```python
from build123d import *

# Parameters (mm, degrees)
SKETCH_1_W           = 29.5
SKETCH_1_H           = 47
EXTRUDE_1_DEPTH      = 70
SKETCH_2_W           = 23.5
SKETCH_2_H           = 44
CUT_EXTRUDE_1_DEPTH  = 70
SKETCH_5_R           = 12
SKETCH_5_R_2         = 3
CUT_EXTRUDE_4_DEPTH  = 70
SKETCH_10_R          = 9
CUT_EXTRUDE_8_DEPTH  = 17
SKETCH_11_W          = 23.5
SKETCH_11_H          = 26.5
SKETCH_11_H_2        = 15
CUT_EXTRUDE_9_DEPTH  = 10
FILLET_2_R           = 5
CUT_EXTRUDE_11_DEPTH = 10
FILLET_3_R           = 5
SKETCH_14_R          = 1.5
CUT_EXTRUDE_12_DEPTH = 10


with BuildPart() as part:
    # 草图1 → 凸台-拉伸1 (new body)
    with BuildSketch(Plane.XY):
        with Locations((14.75, 23.5)):
            Rectangle(SKETCH_1_W, SKETCH_1_H)
    extrude(amount=EXTRUDE_1_DEPTH)

    # 草图2 → 切除-拉伸1 (cut)
    with BuildSketch(Plane.XY.offset(70)):
        with Locations((14.75, 25)):
            Rectangle(SKETCH_2_W, SKETCH_2_H)
    extrude(amount=-CUT_EXTRUDE_1_DEPTH, mode=Mode.SUBTRACT)

    # 草图5 → 切除-拉伸4 (cut)
    with BuildSketch(Plane(origin=(29.5, 0, 0), x_dir=(0, 0, -1), z_dir=(1, 0, 0))):
        with Locations((-17, 32)):
            Circle(SKETCH_5_R)
        with Locations((-62, 32)):
            Circle(SKETCH_5_R_2)
    extrude(amount=-CUT_EXTRUDE_4_DEPTH, mode=Mode.SUBTRACT)

    # 草图10 → 切除-拉伸8 (cut)
    with BuildSketch(Plane(origin=(29.5, 0, 0), x_dir=(0, 0, -1), z_dir=(1, 0, 0))):
        with Locations((-45, 16)):
            Circle(SKETCH_10_R)
    extrude(amount=-CUT_EXTRUDE_8_DEPTH, mode=Mode.SUBTRACT)

    # 草图11 → 切除-拉伸9 (cut)
    with BuildSketch(Plane.XZ):
        with Locations((14.75, 56.75)):
            Rectangle(SKETCH_11_W, SKETCH_11_H)
        with Locations((14.75, 7.5)):
            Rectangle(SKETCH_11_W, SKETCH_11_H_2)
    extrude(amount=-CUT_EXTRUDE_9_DEPTH, mode=Mode.SUBTRACT)

    # 圆角2
    fillet_2_edges = [part.edges().sort_by_distance(p)[0] for p in [
        (1.5, 0, 0),
        (28, 0, 0),
        (28, 0, 70),
        (1.5, 0, 70),
        (3, 1.5, 43.5),
        (26.5, 1.5, 43.5),
    ]]
    fillet(fillet_2_edges, radius=FILLET_2_R)

    # 草图13 → 切除-拉伸11 (cut)
    with BuildSketch(Plane(origin=(3, 0, 0), x_dir=(0, 0, -1), z_dir=(1, 0, 0))):
        Polygon((-15, 0), (-15, 3), (-30, 3), (-56, 47), (0, 47), (0, 0), align=None)
    extrude(amount=-CUT_EXTRUDE_11_DEPTH, mode=Mode.SUBTRACT)

    # 圆角3
    fillet_3_edges = [part.edges().sort_by_distance(p)[0] for p in [
        (28, 47, 70),
        (0, 1.5, 15),
        (1.5, 3, 30),
        (1.5, 47, 56),
        (1.5, 47, 70),
        (28, 47, 0),
        (26.5, 1.5, 15),
    ]]
    fillet(fillet_3_edges, radius=FILLET_3_R)

    # 草图14 → 切除-拉伸12 (cut)
    with BuildSketch(Plane.XZ):
        with Locations(Location((9.75, 35.2, 0), (0, 0, 270))):
            Circle(SKETCH_14_R)
        with Locations(Location((9.75, 23.2, 0), (0, 0, 270))):
            Circle(SKETCH_14_R)
        with Locations(Location((19.75, 23.2, 0), (0, 0, 270))):
            Circle(SKETCH_14_R)
        with Locations(Location((19.75, 35.2, 0), (0, 0, 270))):
            Circle(SKETCH_14_R)
    extrude(amount=-CUT_EXTRUDE_12_DEPTH, mode=Mode.SUBTRACT)


solid = part.part
```
The listing builds one solid part. Answer for the finished solid, in the listing's coordinates (mm). A direction names the side the tool comes from. Coordinates: 2 decimals unless noted, no trailing zeros. Loops run counter-clockwise (first coordinate to the right, second up) from the corner with the lowest first, then second, coordinate; pieces in that order, holes last. Notation, with made-up numbers: (-17, -7) -> (11, -7) arc R16 cw to (11, 4) -> close; hole circle Ø4 at (63.5, 15.25). An arc over 180 degrees is marked (long way). Return JSON: item names as keys, results as strings. Group by question number.
(1) A cutting plane is placed at B-B on x = 19.75. Write down the section's boundary in (y, z).
(2) A cutting plane is placed at D-D on y = 36. Write down the section's boundary in (x, z).
(3) A cutting plane is placed at C-C on z = 35.2. Write down the section's boundary in (x, y), and give its area (3 significant figures).
(4) A cutting plane is placed at A-A on z = 62. Write down the section's boundary in (x, y).
(5) Determine the mould class of faces 6 (the cylindrical face through (28, 46, 2)), 7 (the cylindrical face through (28, 2, 1)), 8 (the cylindrical face through (1.5, 30.2, 64.4)) for opening direction Y: released by +Y, released by -Y, zero draft, split by the parting line, or undercut.
(6) Which of the six approach directions +Z, -Z, +X, -X, +Y, -Y give full straight-line access (tool end or side, diameter ignored) to faces 1 (the cylindrical face through (28, 16, 54)), 2 (the cylindrical face through (21.237, 1.479, 23.395)), 3 (the cylindrical face through (28, 2, 69)), 4 (the flat face through (2, 25, 43)), 5 (the flat face through (15, 1, 43.5))?
(7) Find the intervals of material crossed by probe 1 along X at (y, z) = (1, 35.2); probe 2 along X at (y, z) = (13, 60.5); probe 3 along Y at (x, z) = (27.6, 62), in increasing order. Write a range as from..to.
(8) Given pin 1 Ø13 at (x, z) = (14, 33) entering from +Y; pin 2 Ø2.5 at (x, y) = (16.5, 2) entering from -Z; pin 3 Ø3 at (y, z) = (11, 14.5) entering from -X, each flat-ended and moving along its own axis, determine where each tip first touches the part or whether it passes through.
The answers:
{
 "1": {"outline": "(0, 15) -> (3, 15) -> (3, 21.7) -> (0, 21.7) -> close; (0, 24.7) -> (3, 24.7) -> (3, 33.7) -> (0, 33.7) -> close; (0, 36.7) -> (3, 36.7) -> (3, 43.5) -> (0, 43.5) -> close"},
 "2": {"outline": "(0, 49.5) -> (3, 49.5) -> (3, 70) -> (0, 70) -> close; (26.5, 0) -> (29.5, 0) -> (29.5, 5.69) -> (26.5, 5.69) -> close; (26.5, 28.31) -> (29.5, 28.31) -> (29.5, 70) -> (26.5, 70) -> close"},
 "3": {"outline": "(0, 0) -> (8.25, 0) -> (8.25, 3) -> (3, 3) -> (3, 11.8) -> (0, 11.8) -> close; (11.25, 0) -> (18.25, 0) -> (18.25, 3) -> (11.25, 3) -> close; (21.25, 0) -> (29.5, 0) -> (29.5, 47) -> (26.5, 47) -> (26.5, 3) -> (21.25, 3) -> close", "area": "229 mm^2"},
 "4": {"outline": "(0, 0) -> (3, 0) -> (3, 29) -> (0, 29) -> close; (0, 35) -> (3, 35) -> (3, 47) -> (0, 47) -> close; (26.5, 0) -> (29.5, 0) -> (29.5, 29) -> (26.5, 29) -> close; (26.5, 35) -> (29.5, 35) -> (29.5, 47) -> (26.5, 47) -> close"},
 "5": {"face 6": "released by +Y", "face 7": "released by -Y", "face 8": "undercut"},
 "6": {"face 1": "+X", "face 2": "+Y, -Y", "face 3": "+Z, +X, -X, -Y", "face 4": "-Z, -X, +Y", "face 5": "+Z, +Y, -Y"},
 "7": {"probe 1": "x = 0..8.25, 11.25..18.25, 21.25..29.5", "probe 2": "x = 0..3, 26.5..29.5", "probe 3": "y = 0..29, 35..47"},
 "8": {"pin 1": "stops at y = 3", "pin 2": "stops at z = 15", "pin 3": "stops at x = 26.5"}
}
